Could you check a few things on this model? Use its own coordinates, in mm. Face numbers are marked on the shaded views. A direction names the side the tool comes from. Give positions to 0.01 mm unless a question says otherwise; leave off trailing zeros. Write each loop counter-clockwise with the first axis right and the second up, starting at its lowest first coordinate (ties: lowest second). Pieces come first, ordered by that corner, then holes. Notation, with made-up numbers: (-27.5, 30.5) - (-17.5, 30.5) arc R20 ccw to (-17.5, 36.5) - close; hole circle Ø6 at (45, 61.25). An arc over 180 degrees is marked (long way). Answer in a Markdown table with one row per item.
from build123d import *

# Parameters (mm, degrees)
SKETCH_1_W          = 35
SKETCH_1_H          = 14.4
SKETCH_1_W_2        = 15
SKETCH_1_H_2        = 8.4
EXTRUDE_1_DEPTH     = 3
SKETCH_2_W          = 20
SKETCH_2_H          = 3
CUT_EXTRUDE_1_DEPTH = 1.5
SKETCH_3_R          = 1.6
CUT_EXTRUDE_2_DEPTH = 20
SKETCH_5_R          = 4
CUT_EXTRUDE_4_DEPTH = 10
FILLET_2_R          = 2
SKETCH_6_R          = 0.9
CUT_EXTRUDE_5_DEPTH = 1.5


with BuildPart() as part:
    # 草图1 → 凸台-拉伸1 (new body)
    with BuildSketch(Plane.XY):
        Rectangle(SKETCH_1_W, SKETCH_1_H)
        Rectangle(SKETCH_1_W_2, SKETCH_1_H_2, mode=Mode.SUBTRACT)
    extrude(amount=EXTRUDE_1_DEPTH)

    # 草图2 → 切除-拉伸1 (cut)
    with BuildSketch(Plane.XY.offset(3)):
        Rectangle(SKETCH_2_W, SKETCH_2_H)
    extrude(amount=-CUT_EXTRUDE_1_DEPTH, mode=Mode.SUBTRACT)

    # 草图3 → 切除-拉伸2 (cut)
    with BuildSketch(Plane.XY.offset(3)):
        with Locations((-13, 0)):
            Circle(SKETCH_3_R)
        with Locations((13, 0)):
            Circle(SKETCH_3_R)
    extrude(amount=-CUT_EXTRUDE_2_DEPTH, mode=Mode.SUBTRACT)

    # 草图5 → 切除-拉伸4 (cut)
    with BuildSketch(Plane.XY.offset(3)):
        with Locations((-14.5, 7.2)):
            Circle(SKETCH_5_R)
        with Locations((14.5, 7.2)):
            Circle(SKETCH_5_R)
        with Locations((14.5, -7.2)):
            Circle(SKETCH_5_R)
        with Locations((-14.5, -7.2)):
            Circle(SKETCH_5_R)
    extrude(amount=-CUT_EXTRUDE_4_DEPTH, mode=Mode.SUBTRACT)

    # 圆角2
    fillet_2_edges = [part.edges().sort_by_distance(p)[0] for p in [
        (10.5, -7.2, 1.5),
        (-10.5, -7.2, 1.5),
        (-17.5, 4.554248689, 1.5),
        (10.5, 7.2, 1.5),
        (-17.5, -4.554248689, 1.5),
        (17.5, -4.554248689, 1.5),
        (17.5, 4.554248689, 1.5),
        (-10.5, 7.2, 1.5),
    ]]
    fillet(fillet_2_edges, radius=FILLET_2_R)

    # 草图6 → 切除-拉伸5 (cut)
    with BuildSketch(Plane.XY.offset(3)):
        with Locations((-9.1, 1.5)):
            Circle(SKETCH_6_R)
        with Locations((-9.1, -1.5)):
            Circle(SKETCH_6_R)
        with Locations((9.1, 1.5)):
            Circle(SKETCH_6_R)
        with Locations((9.1, -1.5)):
            Circle(SKETCH_6_R)
    extrude(amount=-CUT_EXTRUDE_5_DEPTH, mode=Mode.SUBTRACT)


solid = part.part
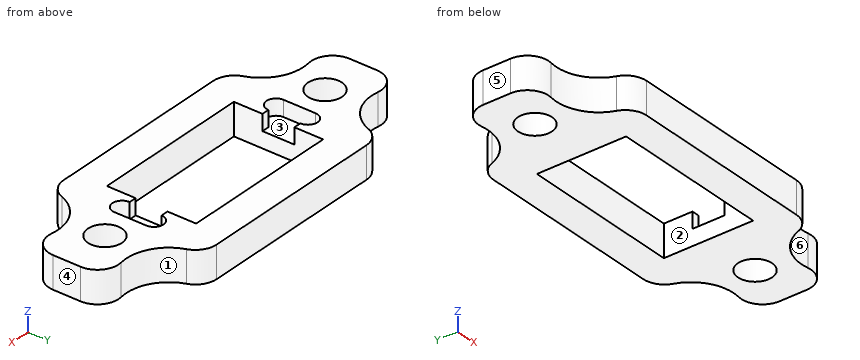
1) Imagine slicing it at C-C (z = 1.1). List the corners of the cut face in (x, y) for me, then the cut area to 3 significant figures.
Check values:
| item | result |
|---|---|
| outline | (-17.5, -1.28) arc R2 ccw to (-15.17, -3.26) arc R4 cw to (-10.73, -5.87) arc R2 ccw to (-8.84, -7.2) - (8.84, -7.2) arc R2 ccw to (10.73, -5.87) arc R4 cw to (15.17, -3.26) arc R2 ccw to (17.5, -1.28) - (17.5, 1.28) arc R2 ccw to (15.17, 3.26) arc R4 cw to (10.73, 5.87) arc R2 ccw to (8.84, 7.2) - (-8.84, 7.2) arc R2 ccw to (-10.73, 5.87) arc R4 cw to (-15.17, 3.26) arc R2 ccw to (-17.5, 1.28) - close; hole circle Ø3.2 at (-13, 0); hole (-7.5, -4.2) - (7.5, -4.2) - (7.5, 4.2) - (-7.5, 4.2) - close; hole circle Ø3.2 at (13, 0) |
| area | 259 mm2 |
2) On a 3-axis mill with a long thin cutter (end or side, diameter ignored), from which of +Z, -Z, +X, -X, +Y, -Y can I reach the whole of each face in a straight line? I mean the marked faces 1, 2 and 3. Say none if no direction works.
Check values:
| item | result |
|---|---|
| face 1 | +Z, -Z, +Y |
| face 2 | +Z, -Z |
| face 3 | +Z |
3) We'd pull the mould along X, two halves only. Please class the marked faces 4, 5 and 6: +X half, -X half, draft (parallel to the pull), parting line (faces both ways), or undercut.
Check values:
| item | result |
|---|---|
| face 4 | +X half |
| face 5 | -X half |
| face 6 | undercut |
4) Imagine slicing it at B-B (x = -6). List the corners of the cut face in (y, z) for me, then the cut area to 3 significant figures.
Check values:
| item | result |
|---|---|
| outline | (-7.2, 0) - (-4.2, 0) - (-4.2, 3) - (-7.2, 3) - close; (4.2, 0) - (7.2, 0) - (7.2, 3) - (4.2, 3) - close |
| area | 18.0 mm2 |
5) Will these pins go through, and if not, where does the flat tip stop? P1, Ø1.5, axis at y = -3, z = 0.5, coming from the -X side; P2, Ø1.2, axis at x = -8.5, y = -0.5, coming from the +Z side; P3, Ø1.9, axis at x = -13, y = 0, coming from the +Z side.
Check values:
| item | result |
|---|---|
| P1 | stops at x = -17.25 |
| P2 | stops at z = 1.5 |
| P3 | passes through |
6) Imagine slicing it at D-D (x = 9.5). List the corners of the cut face in (y, z) for me.
Check values:
| item | result |
|---|---|
| outline | (-7.09, 0) - (7.09, 0) - (7.09, 3) - (2.31, 3) - (2.31, 1.5) - (-2.31, 1.5) - (-2.31, 3) - (-7.09, 3) - close |
7) If I drill on line 1 (Y direction, x = 4, z = 1.1); line 2 (X direction, y = -1.75, z = 2.5); line 3 (X direction, y = -2.75, z = 1.1), over which ranges is the centre line in solid material (lowest first)?
Check values:
| item | result |
|---|---|
| line 1 | y = -7.2 to -4.2, 4.2 to 7.2 |
| line 2 | x = -17.44 to -9.96, -8.24 to -7.5, 7.5 to 8.24, 9.96 to 17.44 |
| line 3 | x = -16.86 to -7.5, 7.5 to 16.86 |
8) Imagine slicing it at A-A (y = 0). List the corners of the cut face in (x, z) for me, then the cut area to 3 significant figures.
Check values:
| item | result |
|---|---|
| outline | (-17.5, 0) - (-14.6, 0) - (-14.6, 3) - (-17.5, 3) - close; (-11.4, 0) - (-7.5, 0) - (-7.5, 1.5) - (-10, 1.5) - (-10, 3) - (-11.4, 3) - close; (7.5, 0) - (11.4, 0) - (11.4, 3) - (10, 3) - (10, 1.5) - (7.5, 1.5) - close; (14.6, 0) - (17.5, 0) - (17.5, 3) - (14.6, 3) - close |
| area | 33.3 mm2 |
